```python
from build123d import *

# Parameters (mm, degrees)
BOSS_EXTRUDE1_DEPTH = 7
SHELL1_T            = -2
FILLET1_R           = 1
SKETCH2_R           = 8.5
BOSS_EXTRUDE2_DEPTH = 1.6
SKETCH3_W           = 4.4
SKETCH3_H           = 2
SKETCH3_W_2         = 2
SKETCH3_H_2         = 4.4
CUT_EXTRUDE1_DEPTH  = 4
FILLET2_R           = 2


with BuildPart() as part:
    # Sketch1 → Boss-Extrude1 (new body)
    with BuildSketch(Plane(origin=(0, 0, 0), x_dir=(1, 0, 0), z_dir=(0, 1, 0))):
        with BuildLine():
            Line((-14, -17), (14, -17))
            ThreePointArc((14, -17), (16.121320344, -16.121320344), (17, -14))
            Line((17, -14), (17, 14))
            ThreePointArc((17, 14), (16.121320344, 16.121320344), (14, 17))
            Line((14, 17), (-14, 17))
            ThreePointArc((-14, 17), (-16.121320344, 16.121320344), (-17, 14))
            Line((-17, 14), (-17, -14))
            ThreePointArc((-17, -14), (-16.121320344, -16.121320344), (-14, -17))
        make_face()
    extrude(amount=BOSS_EXTRUDE1_DEPTH)

    # Shell1
    shell1_openings = [part.faces().sort_by_distance(p)[0] for p in [
        (0, 0, 0),
    ]]
    offset(amount=SHELL1_T, openings=shell1_openings, kind=Kind.INTERSECTION)

    # Fillet1
    fillet1_edges = [part.edges().sort_by_distance(p)[0] for p in [
        (16.121320344, 7, 16.121320344),
        (17, 7, 0),
        (16.121320344, 7, -16.121320344),
        (0, 7, -17),
        (-16.121320344, 7, -16.121320344),
        (-17, 7, 0),
        (-16.121320344, 7, 16.121320344),
        (0, 7, 17),
    ]]
    fillet(fillet1_edges, radius=FILLET1_R)

    # Sketch2 → Boss-Extrude2 (add)
    with BuildSketch(Plane.XZ.offset(-5)):
        with Locations(Location((0, 0, 0), (0, 0, 270))):
            Circle(SKETCH2_R)
    extrude(amount=BOSS_EXTRUDE2_DEPTH)

    # Sketch3 → Cut-Extrude1 (cut)
    with BuildSketch(Plane.XZ):
        with Locations((0, 16)):
            Rectangle(SKETCH3_W, SKETCH3_H)
        with Locations((-16, 0)):
            Rectangle(SKETCH3_W_2, SKETCH3_H_2)
        with Locations((0, -16)):
            Rectangle(SKETCH3_W, SKETCH3_H)
        with Locations((16, 0)):
            Rectangle(SKETCH3_W_2, SKETCH3_H_2)
    extrude(amount=-CUT_EXTRUDE1_DEPTH, mode=Mode.SUBTRACT)

    # Fillet2
    fillet2_edges = [part.edges().sort_by_distance(p)[0] for p in [
        (-15, 2, -2.2),
        (-15, 2, 2.2),
        (-2.2, 2, 15),
        (2.2, 2, 15),
        (15, 2, 2.2),
        (15, 2, -2.2),
        (2.2, 2, -15),
        (-2.2, 2, -15),
    ]]
    fillet(fillet2_edges, radius=FILLET2_R - 0.0001)  # a hair under: the kernel refuses the full size


solid = part.part
```
Part model, mm, in its own coordinate system. A direction names the side the tool comes from. Coordinates: 2 decimals unless noted, no trailing zeros. Order: outer loops, then holes, each group sorted by start corner. A loop starts at its lowest first (then second) coordinate and runs counter-clockwise, first axis right, second up. Notation, with made-up numbers: (43, 33.5) - (62, 33.5) arc R17 cw to (62, 37.5) - close; hole circle Ø4 at (34.25, -20). An arc over 180 degrees is marked (long way). Return JSON: item names as keys, results as strings. Group by question number.
Item 1: Which spindle directions (+Z, -Z, +X, -X, +Y, -Y) get a long thin tool onto all of the face, cutting with end or side? Do faces 4 (the face through (8.428, 4.211, 1.107)), 5 (the face through (0.2, 4.3, -17)). Say none if no direction does.
Item 2: Pin check, flat tips, straight feed: pin 1 (2 mm diameter, centred on x = -16, z = 0.5, fed in from -Y); pin 2 (13.5 mm diameter, centred on x = 2, z = 3.5, fed in from -Y). Stop position of each tip, or through.
Item 3: Cut at D-D (z = -9). List the corners of the cut face in (x, y).
Item 4: Pull direction X, two halves, no side cores. Call faces 1 (the face through (-17, 4.3, -0.2)), 2 (the face through (2.8, 2.03, -15.57)), 3 (the face through (-0.2, 4.3, 17)): pulls with the +X half, pulls with the -X half, needs draft (parallel to the pull), parting line crosses it, or undercut.
Item 5: Cut at C-C (x = 12.5). List the corners of the cut face in (y, z), plus the area to 3 significant figures.
Item 6: Drill centre lines: probe 1 along X at (y, z) = (4.75, 4); probe 2 along Z at (x, y) = (7.5, 1.75); probe 3 along Z at (x, y) = (-3.5, 4.25). Where is each one in solid material? Low to high. Write a range as from..to.
Item 7: Cut at B-B (z = 0). List the corners of the cut face in (x, y), plus the area to 3 significant figures.
Item 8: Cut at A-A (x = 0). List the corners of the cut face in (y, z), plus the area to 3 significant figures.
Check values:
{
 "1": {"face 4": "-Y", "face 5": "-Z, +X, -X, +Y, -Y"},
 "2": {"pin 1": "stops at y = 4", "pin 2": "stops at y = 3.4"},
 "3": {"outline": "(-17, 0) - (-15, 0) - (-15, 5) - (15, 5) - (15, 0) - (17, 0) - (17, 6) arc R1 ccw to (16, 7) - (-16, 7) arc R1 ccw to (-17, 6) - close"},
 "4": {"face 1": "pulls with the -X half", "face 2": "undercut", "face 3": "needs draft"},
 "5": {"outline": "(0, -17) - (6, -17) arc R1 ccw to (7, -16) - (7, 16) arc R1 ccw to (6, 17) - (0, 17) - (0, 15) - (5, 15) - (5, -15) - (0, -15) - close", "area": "87.6 mm2"},
 "6": {"probe 1": "x = -17..-15, -7.5..7.5, 15..17", "probe 2": "z = -17..-15, 15..17", "probe 3": "z = -17..-15, -7.75..7.75, 15..17"},
 "7": {"outline": "(-17, 4) - (-15, 4) - (-15, 5) - (-8.5, 5) - (-8.5, 3.4) - (8.5, 3.4) - (8.5, 5) - (15, 5) - (15, 4) - (17, 4) - (17, 6) arc R1 ccw to (16, 7) - (-16, 7) arc R1 ccw to (-17, 6) - close", "area": "98.8 mm2"},
 "8": {"outline": "(3.4, -8.5) - (5, -8.5) - (5, -15) - (4, -15) - (4, -17) - (6, -17) arc R1 ccw to (7, -16) - (7, 16) arc R1 ccw to (6, 17) - (4, 17) - (4, 15) - (5, 15) - (5, 8.5) - (3.4, 8.5) - close", "area": "98.8 mm2"}
}
